from build123d import *

# Parameters (mm, degrees)
SKETCH_R     = 1.7
SKETCH_R_2   = 1.1
SKETCH_W     = 3
SKETCH_H     = 1.5
PAD_DEPTH    = 6
POCKET_DEPTH = 2.5
SKETCH002_W  = 15.96
SKETCH002_H  = 4.5
SKETCH002_R  = 1.1
PAD001_DEPTH = 3
SKETCH003_W  = 3.7
SKETCH003_H  = 15
PAD002_DEPTH = 6.3
SKETCH004_W  = 15
SKETCH004_H  = 3.5
PAD003_DEPTH = 2.7
SKETCH005_W  = 5
SKETCH005_H  = 9
PAD004_DEPTH = 3


with BuildPart() as part:
    # Sketch → Pad (new body)
    with BuildSketch(Plane.XY):
        Polygon((-20, 7.5), (25, 7.5), (25, -7.5), (-20, -7.5), (-20, -3), (-4.04, -3), (-4.04, 3), (-20, 3), align=None)
        with Locations((5, 0)):
            Circle(SKETCH_R, mode=Mode.SUBTRACT)
        with Locations((13, 0)):
            Circle(SKETCH_R, mode=Mode.SUBTRACT)
        with Locations((-18.25, 5.75)):
            Circle(SKETCH_R_2, mode=Mode.SUBTRACT)
        with Locations((-6.25, 5.75)):
            Circle(SKETCH_R_2, mode=Mode.SUBTRACT)
        with Locations((-18.25, -5.75)):
            Circle(SKETCH_R_2, mode=Mode.SUBTRACT)
        with Locations((-6.25, -5.75)):
            Circle(SKETCH_R_2, mode=Mode.SUBTRACT)
        with Locations((-1.087833, 4)):
            Rectangle(SKETCH_W, SKETCH_H, mode=Mode.SUBTRACT)
        with Locations((-1.087833, -4)):
            Rectangle(SKETCH_W, SKETCH_H, mode=Mode.SUBTRACT)
    extrude(amount=PAD_DEPTH)

    # Sketch001 (on Face24 of Pad) → Pocket (cut)
    with BuildSketch(Plane.XY.offset(6)):
        Polygon((6.6, -2.771281), (8.2, 0), (6.6, 2.771281), (3.4, 2.771281), (1.8, 0), (3.4, -2.771281), align=None)
        Polygon((14.6, -2.771281), (16.2, 0), (14.6, 2.771281), (11.4, 2.771281), (9.8, 0), (11.4, -2.771281), align=None)
    extrude(amount=-POCKET_DEPTH, mode=Mode.SUBTRACT)

    # Sketch002 (on Face5 of Pocket) → Pad001 (join)
    with BuildSketch(Plane.XY.offset(6)):
        with Locations((-12.02, 5.25)):
            Rectangle(SKETCH002_W, SKETCH002_H)
        with Locations((-18.25, 5.75)):
            Circle(SKETCH002_R, mode=Mode.SUBTRACT)
        with Locations((-6.25, 5.75)):
            Circle(SKETCH002_R, mode=Mode.SUBTRACT)
        with Locations((-12.02, -5.25)):
            Rectangle(SKETCH002_W, SKETCH002_H)
        with Locations((-18.25, -5.75)):
            Circle(SKETCH002_R, mode=Mode.SUBTRACT)
        with Locations((-6.25, -5.75)):
            Circle(SKETCH002_R, mode=Mode.SUBTRACT)
    extrude(amount=PAD001_DEPTH)

    # Sketch003 (on Face8 of Pad001) → Pad002 (join)
    with BuildSketch(Plane.XY.offset(6)):
        with Locations((23.15, 0)):
            Rectangle(SKETCH003_W, SKETCH003_H)
    extrude(amount=PAD002_DEPTH)

    # Sketch004 (on Face33 of Pad002) → Pad003 (join)
    with BuildSketch(Plane(origin=(21.3, 0, 0), x_dir=(0, -1, 0), z_dir=(-1, 0, 0))):
        with Locations((0, 10.55)):
            Rectangle(SKETCH004_W, SKETCH004_H)
    extrude(amount=PAD003_DEPTH)

    # Sketch005 (on Face3 of Pad003) → Pad004 (join)
    with BuildSketch(Plane.XZ.offset(-3)):
        with Locations((-17.5, 4.5)):
            Rectangle(SKETCH005_W, SKETCH005_H)
    extrude(amount=PAD004_DEPTH)


solid = part.part
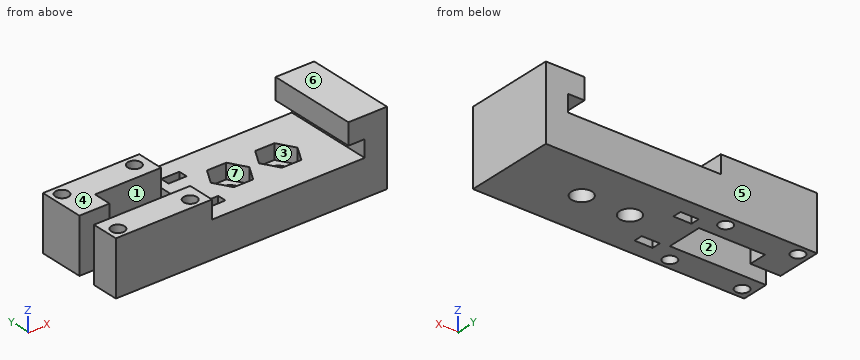
Design review of the part built by this model. Coordinates are the model's own, in mm. Face numbers are marked on the shaded views. A direction names the side the tool comes from. Round coordinates to 2 decimals unless told otherwise and drop trailing zeros. Write each loop counter-clockwise with the first axis right and the second up, starting at its lowest first coordinate (ties: lowest second). Pieces come first, ordered by that corner, then holes.
Item 1: Draft analysis for pull direction Y (two halves, no side actions). For the marked faces 5, 6 and 7, state which applies: released by +Y, released by -Y, zero draft, split by the parting line, or undercut.
Item 2: Consider section A-A on z = 8. Give the boundary of the cut face in (x, y).
Item 3: Consider section B-B on x = 13. Give the boundary of the cut face in (y, z), and give its area (3 significant figures).
Item 4: For the marked faces 1, 2, 3 and 4, list the 3-axis set-ups (+Z, -Z, +X, -X, +Y, -Y) from which the entire face can be reached by the end or side of a thin tool; tool diameter is ignored.
Item 5: Consider section C-C on x = -6.25. Give the boundary of the cut face in (y, z), and give its area (3 significant figures).
Item 6: Wall thickness on L1, parallel to Y at x = -18.25, z = 6.25; L2, parallel to Y at x = -6.25, z = 2.5; L3, parallel to X at y = 3.75, z = 5.5: over which ranges is each line inside the solid? List them lowest first.
Item 7: For pin 1 Ø2 at (y, z) = (-1.5, 6.5) entering from -X; pin 2 Ø2 at (x, y) = (-6.25, 5.75) entering from +Z; pin 3 Ø3.5 at (x, y) = (-12.5, -5) entering from +Z, all flat-tipped, find the tip position at first contact; note any pin that passes through.
Item 8: Consider section D-D on y = -5.75. Give the boundary of the cut face in (x, z).
Check values:
1. face 5: released by +Y
1. face 6: zero draft
1. face 7: undercut
2. outline: (-20, -7.5) - (-4.04, -7.5) - (-4.04, -3) - (-20, -3) - close; (-20, 0) - (-15, 0) - (-15, 3) - (-4.04, 3) - (-4.04, 7.5) - (-20, 7.5) - close; (21.3, -7.5) - (25, -7.5) - (25, 7.5) - (21.3, 7.5) - close; hole circle Ø2.2 at (-18.25, -5.75); hole circle Ø2.2 at (-18.25, 5.75); hole circle Ø2.2 at (-6.25, -5.75); hole circle Ø2.2 at (-6.25, 5.75)
3. outline: (-7.5, 0) - (-1.7, 0) - (-1.7, 3.5) - (-2.77, 3.5) - (-2.77, 6) - (-7.5, 6) - close; (1.7, 0) - (7.5, 0) - (7.5, 6) - (2.77, 6) - (2.77, 3.5) - (1.7, 3.5) - close
3. area: 64.2 mm2
4. face 1: +Z, -Z
4. face 2: +Z, -Z, -X
4. face 3: +Z
4. face 4: +Z, -X, +Y, -Y
5. outline: (-7.5, 0) - (-6.85, 0) - (-6.85, 9) - (-7.5, 9) - close; (-4.65, 0) - (-3, 0) - (-3, 9) - (-4.65, 9) - close; (3, 0) - (4.65, 0) - (4.65, 9) - (3, 9) - close; (6.85, 0) - (7.5, 0) - (7.5, 9) - (6.85, 9) - close
5. area: 41.4 mm2
6. L1: y = -7.5 to -6.85, -4.65 to -3, 0 to 4.65, 6.85 to 7.5
6. L2: y = -7.5 to -6.85, -4.65 to -3, 3 to 4.65, 6.85 to 7.5
6. L3: x = -20 to -2.59, 0.41 to 25
7. pin 1: stops at x = -4.04
7. pin 2: passes through
7. pin 3: stops at z = 9
8. outline: (-20, 0) - (-19.35, 0) - (-19.35, 9) - (-20, 9) - close; (-17.15, 0) - (-7.35, 0) - (-7.35, 9) - (-17.15, 9) - close; (-5.15, 0) - (25, 0) - (25, 12.3) - (18.6, 12.3) - (18.6, 8.8) - (21.3, 8.8) - (21.3, 6) - (-4.04, 6) - (-4.04, 9) - (-5.15, 9) - close
